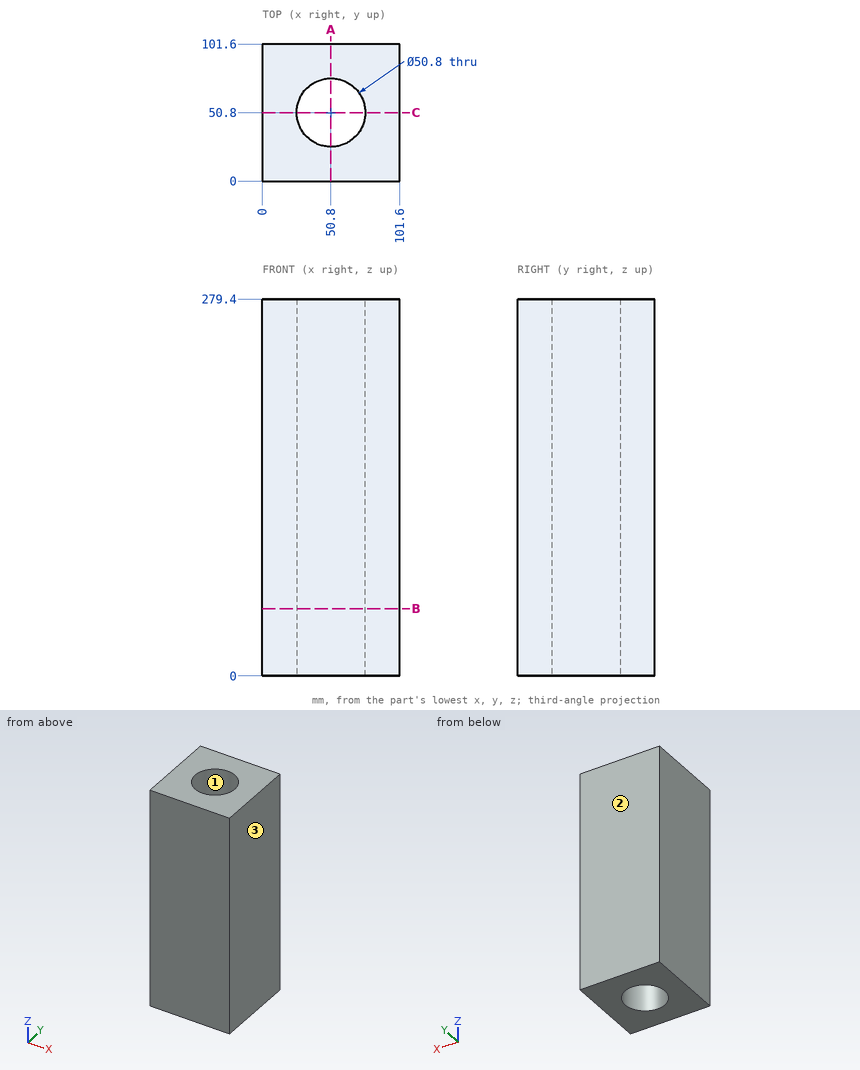
Design review of the part shown in the three views and the two pictorial views. Dimensions are in mm from the part's minimum x, y and z. Give positions to 0.01 mm unless a question says otherwise; leave off trailing zeros. Loops run counter-clockwise (first coordinate to the right, second up) from the corner with the lowest first, then second, coordinate; pieces in that order, holes last. Notation, with made-up numbers: (61, -34.75) -> (96, -34.75) arc R18 ccw to (96, -17.75) -> close; hole circle Ø8 at (59.5, 84.25). An arc over 180 degrees is marked (long way). One line per question, with ' | ' between items.
1) The part is to be moulded in two halves that separate along X. For the marked faces 1, 2 and 3, say which applies: +X half, -X half, draft (parallel to the pull), parting line (faces both ways), or undercut.
Resolved:
face 1: undercut | face 2: draft | face 3: +X half
2) We need section B-B (z = 50). Write out the cut boundary in (x, y), plus the area to 3 significant figures.
Resolved:
outline: (0, 0) -> (101.6, 0) -> (101.6, 101.6) -> (0, 101.6) -> close; hole circle Ø50.8 at (50.8, 50.8) | area: 8,300 mm2
3) We need section A-A (x = 50.8). Write out the cut boundary in (y, z), plus the area to 3 significant figures.
Resolved:
outline: (0, 0) -> (25.4, 0) -> (25.4, 279.4) -> (0, 279.4) -> close; (76.2, 0) -> (101.6, 0) -> (101.6, 279.4) -> (76.2, 279.4) -> close | area: 14,200 mm2
4) To check wall thickness, follow probe 1 along Y at (x, z) = (50.8, 198); probe 2 along X at (y, z) = (73, 124). State the ranges of each line that lie inside material, in increasing order.
Resolved:
probe 1: y = 0 to 25.4, 76.2 to 101.6 | probe 2: x = 0 to 38.46, 63.14 to 101.6
